from build123d import *

# Parameters (mm, degrees)
SKETCH1_W           = 95.25
SKETCH1_H           = 120.65
BOSS_EXTRUDE1_DEPTH = 8.89
SKETCH2_OUTSIDE_W   = 128.044
SKETCH2_OUTSIDE_H   = 153.444
SKETCH2_OUTSIDE_W_2 = 95.25
SKETCH2_OUTSIDE_H_2 = 120.65
SKETCH2_OUTSIDE_R   = 2.38125
CUT_EXTRUDE2_DEPTH  = 9.89
SKETCH3_R           = 7.62
CUT_EXTRUDE3_DEPTH  = 5.08
SKETCH4_R           = 3.3655
CUT_EXTRUDE4_DEPTH  = 4.81
SKETCH5_W           = 50.8
SKETCH5_H           = 22.86
CUT_EXTRUDE5_DEPTH  = 9.89
SKETCH6_W           = 7.62
SKETCH6_H           = 2.54
CUT_EXTRUDE6_DEPTH  = 9.89


with BuildPart() as part:
    # Sketch1 → Boss-Extrude1 (new body)
    with BuildSketch(Plane.XY):
        Rectangle(SKETCH1_W, SKETCH1_H)
    extrude(amount=BOSS_EXTRUDE1_DEPTH)

    # Sketch2 outside → Cut-Extrude2 (cut, through all)
    with BuildSketch(Plane.XY.offset(8.89)):
        Rectangle(SKETCH2_OUTSIDE_W, SKETCH2_OUTSIDE_H)
        Rectangle(SKETCH2_OUTSIDE_W_2, SKETCH2_OUTSIDE_H_2, mode=Mode.SUBTRACT)
        with Locations((-41.275, 52.281666667)):
            Circle(SKETCH2_OUTSIDE_R)
        with Locations((41.275, 52.281666667)):
            Circle(SKETCH2_OUTSIDE_R)
        with Locations((41.275, -52.281666667)):
            Circle(SKETCH2_OUTSIDE_R)
        with Locations((-41.275, -52.281666667)):
            Circle(SKETCH2_OUTSIDE_R)
    extrude(amount=-CUT_EXTRUDE2_DEPTH, mode=Mode.SUBTRACT)

    # Sketch3 → Cut-Extrude3 (cut)
    with BuildSketch(Plane.XY.offset(8.89)):
        with Locations((24.765, 42.545)):
            Circle(SKETCH3_R)
    extrude(amount=-CUT_EXTRUDE3_DEPTH, mode=Mode.SUBTRACT)

    # Sketch4 → Cut-Extrude4 (cut, through all)
    with BuildSketch(Plane.XY.offset(3.81)):
        with Locations((24.765, 42.545)):
            Circle(SKETCH4_R)
    extrude(amount=-CUT_EXTRUDE4_DEPTH, mode=Mode.SUBTRACT)

    # Sketch5 → Cut-Extrude5 (cut, through all)
    with BuildSketch(Plane.XY.offset(8.89)):
        with Locations((-15.113, 18.415)):
            Rectangle(SKETCH5_W, SKETCH5_H)
    extrude(amount=-CUT_EXTRUDE5_DEPTH, mode=Mode.SUBTRACT)

    # Sketch6 → Cut-Extrude6 (cut, through all)
    with BuildSketch(Plane.XY.offset(8.89)):
        with Locations((-43.815, -14.605)):
            Rectangle(SKETCH6_W, SKETCH6_H)
        with Locations((43.815, -14.605)):
            Rectangle(SKETCH6_W, SKETCH6_H)
    extrude(amount=-CUT_EXTRUDE6_DEPTH, mode=Mode.SUBTRACT)


solid = part.part
Work out the finished part from the listing and answer in its coordinate system (mm). A direction names the side the tool comes from. Round coordinates to 2 decimals unless told otherwise and drop trailing zeros. Write each loop counter-clockwise with the first axis right and the second up, starting at its lowest first coordinate (ties: lowest second). Pieces come first, ordered by that corner, then holes. Notation, with made-up numbers: (-30, 47) -> (-4, 47) arc R19 cw to (-4, 70) -> close; hole circle Ø11 at (-4.75, -37). An arc over 180 degrees is marked (long way). Answer as CSV lines item,"result". Start each with the question number.
(1) The part is cut by section D-D, the plane x = 41.5. Give the vertices of the cut face in (y, z) (3 decimals).
(2) The part is cut by section A-A, the plane y = 12.5. Give the vertices of the cut face in (x, z) (3 decimals).
(3) Each of these flat-tipped pins is pushed along its axis until it touches: pin 1 (3 mm diameter, centred on x = -41.28, y = 52.28, fed in from +Z); pin 2 (4.5 mm diameter, centred on x = 25.5, y = 40.5, fed in from +Z). Where does it stop, or does it pass through?
(4) Find the intervals of material crossed by probe 1 along Y at (x, z) = (41, 8.75) (3 decimals); probe 2 along Y at (x, z) = (25, 7.5) (3 decimals); probe 3 along Y at (x, z) = (-14.5, 4.75) (3 decimals), in increasing order.
(5) A tool of negligible diameter and unlimited length cuts with its end or side. For faces 1 (the flat face through (40.005, -15, 5)), 2 (the flat face through (28, 41, 3.81)), 3 (the flat face through (10.287, 18, 5)), from which of +Z, -Z, +X, -X, +Y, -Y can it reach the whole face along a straight path? Write none if from no direction.
(6) The mould has two halves that part along Y. Classify faces 4 (the flat face through (-47.625, -38, 4)), 5 (the flat face through (-1, -60.325, 4)), 6 (the flat face through (-40.005, -15, 5)), 7 (the flat face through (44, -15.875, 5)): +Y half, -Y half, draft (parallel to the pull), parting line (faces both ways), or undercut.
(7) The part is cut by section B-B, the plane x = -9.5. Give the vertices of the cut face in (y, z) (3 decimals).
(8) The part is cut by section C-C, the plane z = 7.5. Give the vertices of the cut face in (x, y) (1 decimal), then the cut area to 3 significant figures.
Output values:
1,outline,"(-60.325, 0) -> (-54.652, 0) -> (-54.652, 8.89) -> (-60.325, 8.89) -> close; (-49.911, 0) -> (-15.875, 0) -> (-15.875, 8.89) -> (-49.911, 8.89) -> close; (-13.335, 0) -> (49.911, 0) -> (49.911, 8.89) -> (-13.335, 8.89) -> close; (54.652, 0) -> (60.325, 0) -> (60.325, 8.89) -> (54.652, 8.89) -> close"
2,outline,"(-47.625, 0) -> (-40.513, 0) -> (-40.513, 8.89) -> (-47.625, 8.89) -> close; (10.287, 0) -> (47.625, 0) -> (47.625, 8.89) -> (10.287, 8.89) -> close"
3,pin 1,"passes through"
3,pin 2,"stops at z = 3.81"
4,probe 1,"y = -60.325 to -54.647, -49.916 to -15.875, -13.335 to 49.916, 54.647 to 60.325"
4,probe 2,"y = -60.325 to 34.929, 50.161 to 60.325"
4,probe 3,"y = -60.325 to 6.985, 29.845 to 60.325"
5,face 1,"+Z, -Z, +X"
5,face 2,"+Z"
5,face 3,"+Z, -Z"
6,face 4,"draft"
6,face 5,"-Y half"
6,face 6,"undercut"
6,face 7,"undercut"
7,outline,"(-60.325, 0) -> (6.985, 0) -> (6.985, 8.89) -> (-60.325, 8.89) -> close; (29.845, 0) -> (60.325, 0) -> (60.325, 8.89) -> (29.845, 8.89) -> close"
8,outline,"(-47.6, -60.3) -> (47.6, -60.3) -> (47.6, -15.9) -> (40, -15.9) -> (40, -13.3) -> (47.6, -13.3) -> (47.6, 60.3) -> (-47.6, 60.3) -> (-47.6, -13.3) -> (-40, -13.3) -> (-40, -15.9) -> (-47.6, -15.9) -> close; hole circle Ø4.8 at (-41.3, -52.3); hole circle Ø4.8 at (-41.3, 52.3); hole (-40.5, 7) -> (10.3, 7) -> (10.3, 29.8) -> (-40.5, 29.8) -> close; hole circle Ø15.2 at (24.8, 42.5); hole circle Ø4.8 at (41.3, -52.3); hole circle Ø4.8 at (41.3, 52.3)"
8,area,"10,000 mm²"
